Geometry check sheet. Reference: drawing and pictorial views, mm from the part's lowest x, y, z. Give positions to 0.01 mm unless a question says otherwise; leave off trailing zeros. Loops run counter-clockwise (first coordinate to the right, second up) from the corner with the lowest first, then second, coordinate; pieces in that order, holes last. Notation, with made-up numbers: (8.25, -37.5) -> (32.25, -37.5) arc R30 cw to (32.25, -13.5) -> close; hole circle Ø10 at (-10.5, 10.25). An arc over 180 degrees is marked (long way). One line per item, written item: value. Start each with the question number.
(1) Scan lines: line 1 along Z through (x, y) = (15, 4.15); line 2 along Z through (x, y) = (35, 6.9); line 3 along Y through (x, z) = (75, 33). Record each from-to range of solid material in increasing order. Write a range as from..to.
(2) Sectioned sample at B-B, the plane z = 15. Record the cut outline in (x, y) (1 decimal).
(3) Sectioned sample at A-A, the plane x = 35. Record the cut outline in (y, z) (1 decimal).
(4) Sectioned sample at C-C, the plane x = 22. Record the cut outline in (y, z) (1 decimal).
(5) Sectioned sample at D-D, the plane z = 53. Record the cut outline in (x, y) (1 decimal), then the cut area to 3 significant figures.
(6) Gauge pin test, flat ends, axial feed: pin 1 Ø2.5 at (y, z) = (9, 16) entering from +X; pin 2 Ø7 at (x, z) = (35, 15) entering from -Y; pin 3 Ø2.5 at (y, z) = (8.5, 9) entering from -X; pin 4 Ø3 at (x, z) = (35, 15) entering from -Y. Record the tip position at first contact, or that the pin passes through.
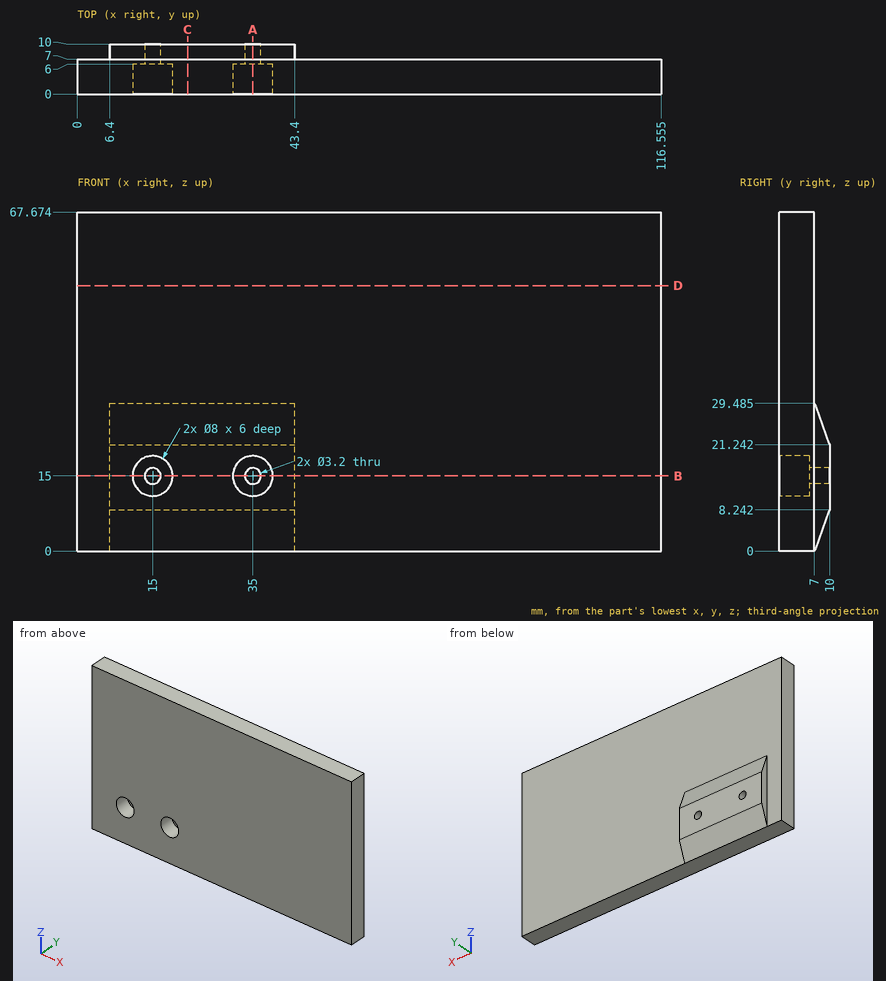
Calculated:
1. line 1: z = 0..11, 19..67.67
1. line 2: z = 0..13.4, 16.6..67.67
1. line 3: y = 0..7
2. outline: (0, 0) -> (11, 0) -> (11, 6) -> (13.4, 6) -> (13.4, 10) -> (6.4, 10) -> (6.4, 7) -> (0, 7) -> close; (16.6, 6) -> (19, 6) -> (19, 0) -> (31, 0) -> (31, 6) -> (33.4, 6) -> (33.4, 10) -> (16.6, 10) -> close; (36.6, 6) -> (39, 6) -> (39, 0) -> (116.6, 0) -> (116.6, 7) -> (43.4, 7) -> (43.4, 10) -> (36.6, 10) -> close
3. outline: (0, 0) -> (7, 0) -> (10, 8.2) -> (10, 13.4) -> (6, 13.4) -> (6, 11) -> (0, 11) -> close; (0, 19) -> (6, 19) -> (6, 16.6) -> (10, 16.6) -> (10, 21.2) -> (7, 29.5) -> (7, 67.7) -> (0, 67.7) -> close
4. outline: (0, 0) -> (7, 0) -> (10, 8.2) -> (10, 21.2) -> (7, 29.5) -> (7, 67.7) -> (0, 67.7) -> close
5. outline: (0, 0) -> (116.6, 0) -> (116.6, 7) -> (0, 7) -> close
5. area: 816 mm2
6. pin 1: stops at x = 43.4
6. pin 2: stops at y = 6
6. pin 3: stops at x = 6.4
6. pin 4: passes through
